Autodesk Inventor part; units mm, degrees
ref_plane "YZ Plane" through (0, 0, 0) normal (1, 0, 0) x (0, 1, 0)
ref_plane "XZ Plane" through (0, 0, 0) normal (0, 1, 0) x (-1, 0, 0)
ref_plane "XY Plane" through (0, 0, 0) normal (0, 0, 1) x (1, 0, 0)
sketch "Sketch1" plane through (0, 0, 0) normal (0, 1, 0) x (-1, 0, 0)
  line L0 (-12.788, 8.8746) -> (7.212, 8.8746)
  line L1 (7.212, 8.8746) -> (7.212, -27.2254)
  line L2 (7.212, -27.2254) -> (-12.788, -27.2254)
  line L3 (-12.788, -27.2254) -> (-12.788, 8.8746)
  point P0 (0, 0)
  dimension "d0" = 20
  dimension "d1" = 36.1
extrude "Extrusion1" add sketch "Sketch1" along normal blind 28
sketch "Sketch2" plane through (0, 0, 0) normal (0, -1, 0) x (1, 0, 0)
  line L0 (-7.212, -27.2254) -> (12.788, -27.2254)
  line L1 (12.788, -27.2254) -> (12.788, 8.8746)
  circle A0 centre (2.788, -8.1254) radius 8.05
  point P0 (0, 0)
  dimension "d4" = 10
  dimension "d5" = 16.1
  dimension "d6" = 19.1
extrude "Extrusion2" cut sketch "Sketch2" against normal blind 30
sketch "Sketch3" plane through (0, 0, 0) normal (0, -1, 0) x (1, 0, 0)
  circle A0 centre (2.788, -8.1254) radius 8.05
  line L0 (12.788, 8.8746) -> (-7.212, 8.8746)
  line L1 (2.038, 8.8746) -> (3.538, 8.8746)
  line L2 (3.538, 8.8746) -> (3.538, -9.1254)
  line L3 (3.538, -9.1254) -> (2.038, -9.1254)
  line L4 (2.038, -9.1254) -> (2.038, 8.8746)
  point P0 (0, 0)
  dimension "d9" = 18
  dimension "d11" = 1.5
  dimension "d12" = 0.75
extrude "Extrusion3" cut sketch "Sketch3" against normal blind 30 contours L2 L3 L4 A0 | A0 L4 L0 L2 picked at (2.8714, -6.11)
sketch "Sketch4" plane through (12.788, 0, -27.2254) normal (0, 0, -1) x (-1, 0, 0)
  line L0 (0, 28) -> (20, 28)
  line L1 (0, 0) -> (0, 28)
  circle A0 centre (10, 14) radius 2.286
  point P0 (12.788, 0)
  dimension "d15" = 14
  dimension "d16" = 10
  dimension "d17" = 4.572
extrude "Extrusion4" cut sketch "Sketch4" against normal blind 10
sketch "Sketch6" plane through (-7.212, 0, -27.2254) normal (-1, 0, 0) x (0, 0, 1)
  line L0 (36.1, 0) -> (0, 0)
  line L1 (36.1, 0) -> (36.1, 28)
  line L2 (0, 28) -> (36.1, 28)
  circle A0 centre (30.1, 6) radius 2.49
  circle A1 centre (30.1, 22) radius 2.49
  point P0 (27.2254, 0)
  dimension "d20" = 6
  dimension "d21" = 6
  dimension "d22" = 4.98
  dimension "d23" = 4.98
  dimension "d24" = 6
  dimension "d25" = 6
extrude "Extrusion5" cut sketch "Sketch6" against normal blind 10
sketch "Sketch7" plane through (12.788, 0, 8.8746) normal (1, 0, 0) x (0, 0, -1)
  circle A0 centre (6, 6) radius 1.725
  circle A1 centre (6, 22) radius 1.725
  line L0 (36.1, 0) -> (0, 0)
  line L1 (0, 28) -> (36.1, 28)
  line L2 (0, 0) -> (0, 28)
  point P0 (8.8746, 0)
  dimension "d28" = 3.45
  dimension "d29" = 3.45
  dimension "d88" = 6
  dimension "d89" = 6
  dimension "d91" = 6
  dimension "d92" = 6
extrude "Extrusion8" cut sketch "Sketch7" against normal blind 10
thread "Thread8"
thread "Thread11"
sketch "Sketch11" plane through (12.788, 0, -27.2254) normal (0, 0, -1) x (-1, 0, 0)
  circle A0 centre (10, 14) radius 2.286
  circle A1 centre (10, 14) radius 0.7841
  circle A2 centre (10, 9) radius 1.0109
  line L0 (10, 18) -> (10, 17) construction
  line L1 (11.0033, 17) -> (11.0033, 18)
  point P0 (12.788, 0)
  point P1 (10, 17.5)
  dimension "d69" = 5
  dimension "d71" = 2.0218
hole "Hole1" at (2.788, 9, -27.2254) direction (0, 0, 1) diameter 2.0218 depth 1.91 tip angle 118
sketch "Sketch13" plane through (12.788, 0, -27.2254) normal (0, 0, -1) x (-1, 0, 0)
  circle A0 centre (10, 9) radius 1.0109
  line L0 (10, 18.5) -> (10, 19.5) construction
  line L1 (11.0109, 18.5) -> (11.0109, 19.5)
  line L2 (8.9891, 19.5) -> (8.9891, 18.5)
  arc A1 (8.9891, 18.5) -> (11.0109, 18.5) centre (10, 18.5) ccw
  arc A2 (11.0109, 19.5) -> (8.9891, 19.5) centre (10, 19.5) ccw
  point P0 (12.788, 0)
  point P1 (10, 19)
  dimension "d81" = 0.5
  dimension "d82" = 2.0218
  dimension "d97" = 10
extrude "Extrusion12" cut sketch "Sketch13" against normal blind 1.91 contours A1 L2 A2 L1
sketch "Sketch15" plane through (-7.212, 0, -27.2254) normal (-1, 0, 0) x (0, 0, 1)
  circle A0 centre (30.1, 22) radius 1.725
  circle A1 centre (30.1, 22) radius 3.9688
  circle A2 centre (30.1, 6) radius 1.725
  circle A3 centre (30.1, 6) radius 3.9687
  point P0 (27.2254, 0)
  point P1 (27.015, 20.5839)
  point P2 (27.015, 23.4161)
  point P3 (27.015, 4.5839)
  point P4 (27.015, 7.4161)
  dimension "d93" = 7.9375
  dimension "d94" = 7.9375
extrude "Extrusion13" cut sketch "Sketch15" against normal blind 4.572 contours A0 | A1 | A2 | A3
sketch "Sketch16" plane through (-7.212, 0, 8.8746) normal (0, 0, 1) x (1, 0, 0)
  circle A0 centre (10, 14) radius 2.286
  circle A1 centre (10, 14) radius 3.9687
  point P0 (7.212, 0)
  dimension "d98" = 7.9375
extrude "Extrusion14" cut sketch "Sketch16" against normal blind 29.622 contours A0 | A1
ref_plane "Work Plane1" through (2.788, 28, 8.8746) normal (1, 0, 0) x (0, 0, -1)
properties part number "Galvo-Holder-PolarisMount_metal_v2"
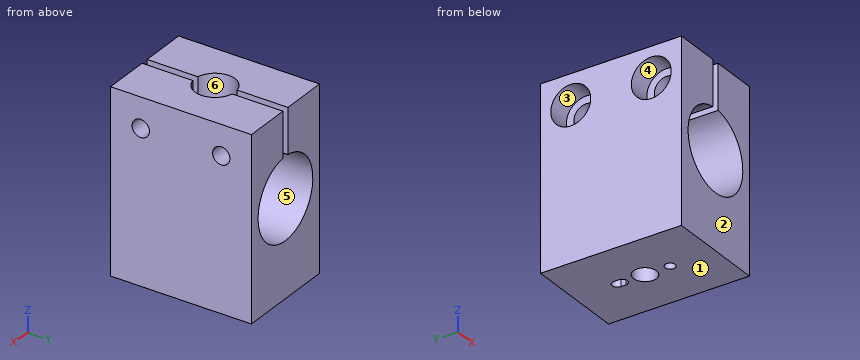
Work out the finished part from the listing and answer in its coordinate system (mm). Face numbers are marked on the shaded views. A direction names the side the tool comes from. Round coordinates to 2 decimals unless told otherwise and drop trailing zeros. Write each loop counter-clockwise with the first axis right and the second up, starting at its lowest first coordinate (ties: lowest second). Pieces come first, ordered by that corner, then holes.
1) Determine the mould class of the marked faces 1, 2 and 3 for opening direction Y: pulls with the +Y half, pulls with the -Y half, needs draft (parallel to the pull), parting line crosses it, or undercut.
2) A cutting plane is placed at B-B on x = 8.5. Determine the outline of the cut face in (y, z) (3 decimals).
3) Which of the six approach directions +Z, -Z, +X, -X, +Y, -Y give full straight-line access (tool end or side, diameter ignored) to the marked faces 4, 5 and 6?
4) A cutting plane is placed at C-C on y = 14. Determine the outline of the cut face in (x, z).
5) A cutting plane is placed at D-D on z = -10. Determine the outline of the cut face in (x, y), and give its area (3 significant figures).
6) Consider probe 1 along Z at (x, y) = (4.5, 20.5); probe 2 along X at (y, z) = (20, 6); probe 3 along X at (y, z) = (9, -26.7). Determine where each line is inside the solid, lowest interval first.
7) Flat-ended cylindrical pins translate along their axes: P1, Ø3, axis at y = 6, z = 2.87, coming from the -X side; P2, Ø7.5, axis at x = 2.788, y = 14, coming from the +Z side; P3, Ø1.8, axis at x = 2.788, y = 9, coming from the -Z side. Find the tip coordinate at first contact, or state that the pin passes through.
8) A cutting plane is placed at A-A on y = 22. Determine the outline of the cut face in (x, z).
Entries:
1. face 1: needs draft
1. face 2: pulls with the -Y half
1. face 3: undercut
2. outline: (0, -27.225) - (28, -27.225) - (28, -13.798) - (0, -13.798) - close; (0, -2.453) - (28, -2.453) - (28, 8.875) - (0, 8.875) - close; hole circle Ø3.45 at (6, 2.875); hole circle Ø3.45 at (22, 2.875)
3. face 4: -X
3. face 5: +Y, -Y
3. face 6: +Z
4. outline: (-7.21, -27.23) - (0.5, -27.23) - (0.5, -20.75) - (-1.18, -20.75) - (-1.18, -15.13) arc R8.05 cw to (-1.18, -1.12) - (-1.18, 8.87) - (-7.21, 8.87) - close; (5.07, -27.23) - (12.79, -27.23) - (12.79, 8.87) - (6.76, 8.87) - (6.76, -1.12) arc R8.05 cw to (6.76, -15.13) - (6.76, -20.75) - (5.07, -20.75) - close
5. outline: (-7.21, 0) - (-5.04, 0) - (-5.04, 28) - (-7.21, 28) - close; (10.62, 0) - (12.79, 0) - (12.79, 28) - (10.62, 28) - close
5. area: 122 mm2
6. probe 1: z = -27.23 to -15.99, -0.26 to 2.02, 3.73 to 8.87
6. probe 2: x = -2.64 to 2.04, 3.54 to 12.79
6. probe 3: x = -7.21 to 1.78, 3.8 to 12.79
7. P1: passes through
7. P2: stops at z = -20.75
7. P3: stops at z = -25.25
8. outline: (-7.21, -27.23) - (12.79, -27.23) - (12.79, 1.15) - (3.54, 1.15) - (3.54, -0.11) arc R8.05 cw (long way) to (2.04, -0.11) - (2.04, 0.38) - (-2.64, 0.38) - (-2.64, -1.09) - (-7.21, -1.09) - close; (-7.21, 6.84) - (-2.64, 6.84) - (-2.64, 5.36) - (2.04, 5.36) - (2.04, 8.87) - (-7.21, 8.87) - close; (3.54, 4.6) - (12.79, 4.6) - (12.79, 8.87) - (3.54, 8.87) - close
